Check sheet for the modelled part. Datum: model origin and axes. Units: mm. A direction names the side the tool comes from. Give positions to 0.01 mm unless a question says otherwise; leave off trailing zeros. Loops run counter-clockwise (first coordinate to the right, second up) from the corner with the lowest first, then second, coordinate; pieces in that order, holes last.
Autodesk Fusion 360 part; units mm, degrees
sketch "Sketch1" plane through (0, 0, 0) normal (0, 0, 1) x (1, 0, 0)
  circle A0 centre (0, 28) radius 5
  circle A1 centre (-28, 0) radius 5
  circle A2 centre (0, -28) radius 5
  line L0 (0, 17.5) -> (35.9687, 17.5)
  line L1 (0, -17.5) -> (35.9687, -17.5)
  arc A3 (35.9687, 17.5) -> (35.9687, -17.5) centre (0, 0) ccw
  arc A4 (0, 17.5) -> (0, -17.5) centre (0, 0) ccw
  dimension "d1" = 80
  dimension "d2" = 35
  dimension "d3" = 28
  dimension "d4" = 10
  dimension "d6" = 180
extrude "Extrude1" add sketch "Sketch1" along normal blind 5
(1) Section check C-C on y = -10.5. Record the boundary of the cut face in (x, z), plus the area to 3 significant figures.
(2) Material ranges on line 1 (Y direction, x = 0, z = 1.45); line 2 (Y direction, x = -2.5, z = 4.3); line 3 (Y direction, x = 7.5, z = 3.95), recorded low to high.
(3) Section check D-D on x = -34. Record the boundary of the cut face in (y, z), plus the area to 3 significant figures.
(4) Access from +Z, -Z, +X, -X, +Y, -Y to the whole of each face (thin tool, end or side, straight path). Record for faces 1 (the face through (18, -17.5, 2)), 2 (the face through (-1.08, 32.88, 2.46)).
(5) Section check A-A on y = 0. Record the boundary of the cut face in (x, z), plus the area to 3 significant figures.
(6) Release check for a two-part mould opening along X. For faces 3 (the face through (-39.97, -1.51, 2.46)), 4 (the face through (18, 17.5, 2)), 5 (the face through (-33, 0, 2)) record: pulls with the +X half, pulls with the -X half, needs draft (parallel to the pull), parting line crosses it, or undercut.
(7) Section check B-B on x = 7.5. Record the boundary of the cut face in (y, z), plus the area to 3 significant figures.
(8) Gauge pin test, flat ends, axial feed: pin 1 Ø13 at (x, y) = (-28, 0) entering from +Z; pin 2 Ø2.5 at (x, z) = (13.5, 1.5) entering from +Y; pin 3 Ø1.5 at (y, z) = (-5, 4.5) entering from -X; pin 4 Ø3 at (y, z) = (8, 1) entering from -X. Record the tip position at first contact, or that the pin passes through.
Computed values:
1. outline: (-38.6, 0) - (-14, 0) - (-14, 5) - (-38.6, 5) - close
1. area: 123 mm2
2. line 1: y = -40 to -33, -23 to -17.5, 17.5 to 23, 33 to 40
2. line 2: y = -39.92 to -32.33, -23.67 to -17.32, 17.32 to 23.67, 32.33 to 39.92
2. line 3: y = -39.29 to -17.5, 17.5 to 39.29
3. outline: (-21.07, 0) - (21.07, 0) - (21.07, 5) - (-21.07, 5) - close
3. area: 211 mm2
4. face 1: +Z, -Z, +X
4. face 2: +Z, -Z
5. outline: (-40, 0) - (-33, 0) - (-33, 5) - (-40, 5) - close; (-23, 0) - (-17.5, 0) - (-17.5, 5) - (-23, 5) - close
5. area: 62.5 mm2
6. face 3: parting line crosses it
6. face 4: needs draft
6. face 5: undercut
7. outline: (-39.29, 0) - (-17.5, 0) - (-17.5, 5) - (-39.29, 5) - close; (17.5, 0) - (39.29, 0) - (39.29, 5) - (17.5, 5) - close
7. area: 218 mm2
8. pin 1: stops at z = 5
8. pin 2: stops at y = 38.08
8. pin 3: stops at x = -39.77
8. pin 4: stops at x = -39.47
